Verification items for the finished model (mm, model axes). A direction names the side the tool comes from. Round coordinates to 2 decimals unless told otherwise and drop trailing zeros. Order: outer loops, then holes, each group sorted by start corner. A loop starts at its lowest first (then second) coordinate and runs counter-clockwise, first axis right, second up. Notation, with made-up numbers: (40, -26.5) -> (64, -26.5) arc R15 ccw to (64, -3.5) -> close; hole circle Ø4 at (57, 86.5). An arc over 180 degrees is marked (long way). Put each result on its own line as item: value.
```python
from build123d import *

# Parameters (mm, degrees)
SKETCH2_R           = 12
SKETCH2_R_2         = 4
BOSS_EXTRUDE1_DEPTH = 5


with BuildPart() as part:
    # Sketch2 → Boss-Extrude1 (new body)
    # profile 1 of 5: a face of its own
    with BuildSketch(Plane.XY):
        with BuildLine():
            ThreePointArc((0, 101.058278507), (-14.142135624, 95.200414131), (-20, 81.058278507))
            Line((-20, 81.058278507), (-8.978854785, 7.961166168))
            ThreePointArc((-8.978854785, 7.961166168), (0.973561331, 11.96044223), (10.148177695, 6.404255575))
            Line((10.148177695, 6.404255575), (37.612146598, 43.558278507))
            ThreePointArc((37.612146598, 43.558278507), (43.529493891, 58.89995601), (40.768147941, 75.109738122))
            ThreePointArc((40.768147941, 75.109738122), (24.162825966, 94.020863263), (0, 101.058278507))
        make_face()
    # profile 2 of 5: a face of its own
    with BuildSketch(Plane.XY):
        with BuildLine():
            ThreePointArc((-7.914553223, -9.019969361), (-11.976499885, -0.750633402), (-8.978854785, 7.961166168))
            Line((-8.978854785, 7.961166168), (-42.420167513, 37.612146598))
            ThreePointArc((-42.420167513, 37.612146598), (-57.761845016, 43.529493891), (-73.971627128, 40.768147941))
            ThreePointArc((-73.971627128, 40.768147941), (-92.882752269, 24.162825966), (-99.920167513, 0))
            ThreePointArc((-99.920167513, 0), (-94.062303137, -14.142135624), (-79.920167513, -20))
            Line((-79.920167513, -20), (-7.914553223, -9.019969361))
        make_face()
    # profile 3 of 5: a face of its own
    with BuildSketch(Plane.XY):
        with BuildLine():
            Line((80, 20), (10.148177695, 6.404255575))
            ThreePointArc((10.148177695, 6.404255575), (11.527752, 3.333306741), (12, 0))
            ThreePointArc((12, 0), (11.221304846, -4.252330837), (8.986280409, -7.952783438))
            Line((8.986280409, -7.952783438), (42.5, -37.612146598))
            ThreePointArc((42.5, -37.612146598), (57.841677503, -43.529493891), (74.051459615, -40.768147941))
            ThreePointArc((74.051459615, -40.768147941), (92.962584756, -24.162825966), (100, 0))
            ThreePointArc((100, 0), (94.142135624, 14.142135624), (80, 20))
        make_face()
    # profile 4 of 5: a face of its own
    with BuildSketch(Plane.XY):
        with BuildLine():
            ThreePointArc((8.986280409, -7.952783438), (0.756221686, -11.976148327), (-7.914553223, -9.019969361))
            Line((-7.914553223, -9.019969361), (-37.612146598, -42.865389918))
            ThreePointArc((-37.612146598, -42.865389918), (-43.529493891, -58.207067421), (-40.768147941, -74.416849533))
            ThreePointArc((-40.768147941, -74.416849533), (-24.162825966, -93.327974674), (0, -100.365389918))
            ThreePointArc((0, -100.365389918), (14.142135624, -94.507525542), (20, -80.365389918))
            Line((20, -80.365389918), (8.986280409, -7.952783438))
        make_face()
    # profile 5 of 5: a face of its own
    with BuildSketch(Plane.XY):
        Circle(SKETCH2_R)
        Circle(SKETCH2_R_2, mode=Mode.SUBTRACT)
    extrude(amount=BOSS_EXTRUDE1_DEPTH)


solid = part.part
```
Item 1: Tool access check on faces 5 (the face through (23.688, 24.721, 2.465)), 6 (the face through (21, 2, 0)). Record the directions out of +Z, -Z, +X, -X, +Y, -Y that give a thin tool (end or side, any length) a straight path to the whole face; none if there is none.
Geometry check:
face 5: +Z, -Z
face 6: -Z, +X, -X, +Y, -Y
Item 2: Sectioned sample at A-A, the plane z = 2.1. Record the boundary of the cut face in (x, y), then the cut area to 3 significant figures.
Geometry check:
outline: (-99.92, 0) arc R20 ccw to (-79.92, -20) -> (-7.91, -9.02) -> (-37.61, -42.87) arc R31 ccw to (-40.77, -74.42) arc R45 ccw to (0, -100.37) arc R20 ccw to (20, -80.37) -> (8.99, -7.95) -> (42.5, -37.61) arc R31 ccw to (74.05, -40.77) arc R45 ccw to (100, 0) arc R20 ccw to (80, 20) -> (10.15, 6.4) -> (37.61, 43.56) arc R31 ccw to (40.77, 75.11) arc R45 ccw to (0, 101.06) arc R20 ccw to (-20, 81.06) -> (-8.98, 7.96) -> (-42.42, 37.61) arc R31 ccw to (-73.97, 40.77) arc R45 ccw to start; hole circle Ø8 at (0, 0)
area: 17,100 mm2
Item 3: Sectioned sample at C-C, the plane x = -12. Record the boundary of the cut face in (y, z), then the cut area to 3 significant figures.
Geometry check:
outline: (-98.74, 0) -> (-13.68, 0) -> (-13.68, 5) -> (-98.74, 5) -> close; (-9.64, 0) -> (10.64, 0) -> (10.64, 5) -> (-9.64, 5) -> close; (28, 0) -> (97.06, 0) -> (97.06, 5) -> (28, 5) -> close
area: 872 mm2
Item 4: Release check for a two-part mould opening along Y. For faces 1 (the face through (21, 2, 5)), 2 (the face through (24.46, 93.83, 2.46)), 3 (the face through (45.563, 13.297, 2.465)), 4 (the face through (13.99, -94.66, 2.46)) record: pulls with the +Y half, pulls with the -Y half, needs draft (parallel to the pull), parting line crosses it, or undercut.
Geometry check:
face 1: needs draft
face 2: pulls with the +Y half
face 3: undercut
face 4: pulls with the -Y half
Item 5: Depth check by flat-ended pin: pin 1 Ø2 at (x, y) = (-48.5, 23) entering from -Z; pin 2 Ø2 at (y, z) = (-28.5, 0.5) entering from +X; pin 3 Ø7 at (x, y) = (0, 0) entering from -Z. Enter the tip coordinate at first touch or a pass-through.
Geometry check:
pin 1: z = 0
pin 2: x = 90.62
pin 3: through
Item 6: Material ranges on line 1 along Y through (x, z) = (-30.5, 2.6); line 2 along X through (y, z) = (-29, 4.3); line 3 along Y through (x, z) = (-6.5, 4.5), recorded low to high.
Geometry check:
line 1: -88.45 to -34.76, -12.46 to 27.04
line 2: -25.45 to 12.19, 32.77 to 89.41
line 3: -99.89 to 99.97
Item 7: Sectioned sample at B-B, the plane x = 27.5. Record the boundary of the cut face in (y, z).
Geometry check:
outline: (-24.34, 0) -> (9.78, 0) -> (9.78, 5) -> (-24.34, 5) -> close; (29.88, 0) -> (91.68, 0) -> (91.68, 5) -> (29.88, 5) -> close
Item 8: Sectioned sample at D-D, the plane y = 53. Record the boundary of the cut face in (x, z).
Geometry check:
outline: (-15.77, 0) -> (42.35, 0) -> (42.35, 5) -> (-15.77, 5) -> close
